Geometry: final body of the model. Coordinates: model frame, mm. A direction names the side the tool comes from. Give positions to 0.01 mm unless a question says otherwise; leave off trailing zeros.
Autodesk Fusion 360 part; units mm, degrees
sketch "Sketch1" plane through (0, 0, 0) normal (1, 0, 0) x (0, 1, 0)
  spline S0 degree 5 poles (-20, 0) (-22.7257, -0.3253) (-28.0984, -1.0502) (-35.9212, -2.3607) (-45.8716, -4.5618) (-57.453, -8.1224) (-68.0948, -12.571) (-77.709, -17.9907) (-86.2289, -24.4443) (-93.6692, -31.9182) (-100.0996, -40.3463) (-104.4963, -47.7952) (-107.3992, -53.7549) (-109.1618, -57.8911) (-110, -60) knots 0 0 0 0 0 0 0.1 0.2 0.3 0.4 0.5 0.6 0.7 0.8 0.9 1 1 1 1 1 1
  spline S1 degree 3 poles (-19.6445, -2.9789) (-34.008, -4.693) (-47.0407, -7.6194) (-58.39, -11.9827) (-67.6436, -15.5402) (-75.7205, -20.0828) (-82.5658, -25.7517) (-91.5958, -33.2299) (-98.5876, -42.6658) (-103.9793, -53.7643) (-105.1319, -56.1368) (-106.2094, -58.5851) (-107.2121, -61.108) knots 0 0 0 0 0.320426 0.320426 0.320426 0.581685 0.581685 0.581685 0.926327 0.926327 0.926327 1 1 1 1
  line L0 (0, 0) -> (0, -2.9702)
  line L1 (-110, -60) -> (-106.765, -60)
  line L2 (-20, 0) -> (0, 0)
  line L3 (-19.6445, -2.9789) -> (0, -2.9702)
  point P0 (-80, -20)
  dimension "d1" = 110
  dimension "d2" = 60
  dimension "d3" = 80
  dimension "d4" = 20
  dimension "d5" = -3
  dimension "d18" = 20
revolve "Revolve1" add sketch "Sketch1" angle 360 about axis through (0, 0, 1.75) along (0, 0, 1)
ref_plane "WorkPlane1" through (0, 0, -2) normal (0, 0, 1) x (1, 0, 0)
sketch "Sketch2" plane through (0, 0, -2) normal (0, 0, 1) x (1, 0, 0)
  circle A0 centre (0, 0) radius 22.5
  dimension "d7" = 45
extrude "Extrude1" add sketch "Sketch2" against normal blind 25
sketch "Sketch3" plane through (0, 0, -27) normal (0, 0, -1) x (1, 0, 0)
  circle A0 centre (0, 0) radius 22.5
  circle A1 centre (10.6066, -10.6066) radius 2.05
  circle A2 centre (3.8823, 14.4889) radius 2.05
  circle A3 centre (-14.4889, -3.8823) radius 2.05
  line L0 (0, 0) -> (10.6066, -10.6066) construction
  dimension "d10" = 4.1
  dimension "d14" = 360
  dimension "d19" = 15
extrude "Extrude2" cut sketch "Sketch3" against normal blind 15 contours A1 | A2 | A3
sketch "Sketch4" plane through (0, 0, -27) normal (0, 0, -1) x (1, 0, 0)
  circle A0 centre (10.6066, -10.6066) radius 2.05
  circle A1 centre (-14.4889, -3.8823) radius 2.05
  circle A2 centre (3.8823, 14.4889) radius 2.05
  circle A3 centre (0, 0) radius 22.5
  circle A4 centre (0, 0) radius 5
  dimension "d20" = 10
extrude "Extrude3" cut sketch "Sketch4" against normal blind 5 contours A4
Item 1: Draft query along Y for faces 1 (the face through (0, 0, 0)), 2 (the face through (0, 0, -22)). Return one class per face: +Y half, -Y half, draft (parallel to the pull), parting line (faces both ways), or undercut.
Values follow:
face 1: draft
face 2: undercut
Item 2: Pin query (flat end, axial travel): pin 1 (1.2 mm diameter, centred on x = 4.5, y = -14, fed in from -Z); pin 2 (11 mm diameter, centred on x = 0, y = -0.5, fed in from -Z); pin 3 (1.5 mm diameter, centred on y = -2.5, z = -29, fed in from +X). Return the tip coordinate at first contact, or that it passes through.
Values follow:
pin 1: stops at z = -12
pin 2: stops at z = -27
pin 3: stops at x = 91.19
Item 3: Ray query, probe 1 along X at (y, z) = (0, -25.65); probe 2 along Y at (x, z) = (-15, -21.5); probe 3 along X at (y, z) = (0, -24.15). Return the intervals inside material, ascending.
Values follow:
probe 1: x = -87.03 to -82.44, -22.5 to -5, 5 to 22.5, 82.44 to 87.03
probe 2: y = -80.65 to -75.42, -16.77 to 1.9, 5.87 to 16.77, 75.42 to 80.65
probe 3: x = -85.32 to -80.56, -22.5 to -5, 5 to 22.5, 80.56 to 85.32
Item 4: Section query A-A on z = -16. Give the number of separate pieces and of enclosed holes in the cut face, plus the area to 3 significant figures.
Values follow:
separate pieces: 2
enclosed holes: 4
area: 4,350 mm2
Item 5: Set-up query: faces 3 (the face through (-0.3, 5.3, -27)), 4 (the face through (58, 90, -60)). Return all of +Z, -Z, +X, -X, +Y, -Y with unobstructed straight access to the full face (end or side cutting, diameter ignored); none if empty.
Values follow:
face 3: -Z
face 4: -Z, +X, -X, +Y, -Y
